Build history of the part. All positions in model axes, mm. A direction names the side the tool comes from. Round coordinates to 2 decimals unless told otherwise and drop trailing zeros. Order: outer loops, then holes, each group sorted by start corner. A loop starts at its lowest first (then second) coordinate and runs counter-clockwise, first axis right, second up. Notation, with made-up numbers: (68.5, 69) -> (88.5, 69) arc R13 cw to (88.5, 91) -> close; hole circle Ø6 at (-34.75, 60). An arc over 180 degrees is marked (long way). Write item = value, one per line.
from build123d import *

# Parameters (mm, degrees)
SKETCH_R             = 50
PAD_DEPTH            = 20
FILLET_R             = 5
SKETCH001_R          = 47
POCKET_DEPTH         = 17
FILLET001_R          = 5
SKETCH002_R          = 2
POCKET001_DEPTH      = 5
SKETCH003_W          = 7
SKETCH003_H          = 5
POCKET002_DEPTH      = 50.001
POCKET002_DEPTH_BACK = -50.001


with BuildPart() as part:
    # Sketch → Pad (new body)
    with BuildSketch(Plane.XY):
        Circle(SKETCH_R)
    extrude(amount=PAD_DEPTH)

    # Fillet
    fillet_edges = [part.edges().sort_by_distance(p)[0] for p in [
        (-50, 0, 0),
    ]]
    fillet(fillet_edges, radius=FILLET_R)

    # Sketch001 (on Face3 of Fillet) → Pocket (cut)
    with BuildSketch(Plane.XY.offset(20)):
        Circle(SKETCH001_R)
    extrude(amount=-POCKET_DEPTH, mode=Mode.SUBTRACT)

    # Fillet001
    fillet001_edges = [part.edges().sort_by_distance(p)[0] for p in [
        (-47, 0, 3),
    ]]
    fillet(fillet001_edges, radius=FILLET001_R)

    # Sketch002 (on Face4 of Fillet001) → Pocket001 (cut)
    with BuildSketch(Plane.XY.offset(3)):
        with Locations((-7.5, 0)):
            Circle(SKETCH002_R)
        with Locations((7.5, 0)):
            Circle(SKETCH002_R)
    extrude(amount=-POCKET001_DEPTH, mode=Mode.SUBTRACT)

    # Sketch003 (on DatumPlane) → Pocket002 (cut, two sides)
    with BuildSketch(Plane(origin=(0, 0, 5), x_dir=(0, 0, -1), z_dir=(0, 1, 0))) as pocket002_sk:
        with Locations((-11.5, 0)):
            Rectangle(SKETCH003_W, SKETCH003_H)
    extrude(amount=-POCKET002_DEPTH, mode=Mode.SUBTRACT)
    extrude(pocket002_sk.sketch, amount=-POCKET002_DEPTH_BACK, mode=Mode.SUBTRACT)


solid = part.part
Q1. Probe probe 1 along X at (y, z) = (1.5, 9); probe 2 along Z at (x, y) = (-31, 12); probe 3 along Y at (x, z) = (0, 10.5). List the from-to ranges inside material, lowest first.
Check values:
probe_1 = -49.98 to -46.98, 46.98 to 49.98
probe_2 = 0 to 3
probe_3 = -50 to -47, 47 to 50
Q2. Which spindle directions (+Z, -Z, +X, -X, +Y, -Y) get a long thin tool onto all of the face, cutting with end or side? Do faces 1 (the face through (-1, 1, 3)), 2 (the face through (0, 48, 13)), 3 (the face through (-1, 1, 0)). Say none if no direction does.
Check values:
face_1 = +Z
face_2 = +Z, +Y, -Y
face_3 = -Z, +X, -X, +Y, -Y
Q3. Flat gauge pins, fed straight in: pin 1 (10 mm diameter, centred on x = 14, z = 15.5, fed in from +Y); pin 2 (2.5 mm diameter, centred on x = 7.5, y = 0, fed in from -Z); pin 3 (6 mm diameter, centred on x = 9, z = 4.5, fed in from +Y); pin 4 (0.9 mm diameter, centred on x = -1, y = -48.5, fed in from +Z). Where does each tip first touch, or does it go through?
Check values:
pin_1 = 49.18
pin_2 = through
pin_3 = 49.63
pin_4 = 13
Q4. Cut at B-B, the plane y = 0. List the corners of the cut face in (x, z), and give its area (3 significant figures).
Check values:
outline = (-50, 5) arc R5 ccw to (-45, 0) -> (-9.5, 0) -> (-9.5, 3) -> (-42, 3) arc R5 cw to (-47, 8) -> (-47, 20) -> (-50, 20) -> close; (-5.5, 0) -> (5.5, 0) -> (5.5, 3) -> (-5.5, 3) -> close; (9.5, 0) -> (45, 0) arc R5 ccw to (50, 5) -> (50, 20) -> (47, 20) -> (47, 8) arc R5 cw to (42, 3) -> (9.5, 3) -> close
area = 378 mm²
Q5. Mould opens along Y. For faces 4 (the face through (47.69, 15.02, 12.4)), 5 (the face through (5.502, 0.088, 1.521)), 6 (the face through (2.5, 48, 17)) say: released by +Y, released by -Y, zero draft, split by the parting line, or undercut.
Check values:
face_4 = split by the parting line
face_5 = undercut
face_6 = zero draft
Q6. Cut at D-D, the plane z = 10.25. List the corners of the cut face in (x, y).
Check values:
outline = circle Ø100 at (0, 0); hole circle Ø94 at (0, 0)
Q7. Cut at C-C, the plane x = 0. List the corners of the cut face in (y, z), and give its area (3 significant figures).
Check values:
outline = (-50, 5) arc R5 ccw to (-45, 0) -> (45, 0) arc R5 ccw to (50, 5) -> (50, 13) -> (47, 13) -> (47, 8) arc R5 cw to (42, 3) -> (-42, 3) arc R5 cw to (-47, 8) -> (-47, 13) -> (-50, 13) -> close
area = 360 mm²
